from build123d import *

# Parameters (mm, degrees)
BOSS_EXTRUDE1_DEPTH = 12.7
SKETCH2_R           = 2.2479
CUT_EXTRUDE1_DEPTH  = 6.35
SKETCH3_W           = 25.4
SKETCH3_H           = 6.35
CUT_EXTRUDE2_DEPTH  = 6.35


with BuildPart() as part:
    # Sketch1 → Boss-Extrude1 (new body)
    with BuildSketch(Plane(origin=(0, 0, 0), x_dir=(1, 0, 0), z_dir=(0, 1, 0))):
        with BuildLine():
            ThreePointArc((0, -2.2479), (-2.2479, 0), (0, 2.2479))
            Line((0, 2.2479), (0, 3.175))
            ThreePointArc((0, 3.175), (-3.175, 0), (0, -3.175))
            Line((0, -3.175), (0, -2.2479))
        make_face()
        with BuildLine():
            ThreePointArc((0, -3.175), (-3.175, 0), (0, 3.175))
            Line((0, 3.175), (5.499261314, 3.175))
            ThreePointArc((5.499261314, 3.175), (-6.35, 0), (5.499261314, -3.175))
            Line((5.499261314, -3.175), (0, -3.175))
        make_face()
        with BuildLine():
            ThreePointArc((0, 2.2479), (1.589505333, 1.589505333), (2.2479, 0))
            Line((2.2479, 0), (3.175, 0))
            ThreePointArc((3.175, 0), (2.24506403, 2.24506403), (0, 3.175))
            Line((0, 3.175), (0, 2.2479))
        make_face()
        with BuildLine():
            Line((3.175, 0), (2.2479, 0))
            ThreePointArc((2.2479, 0), (1.589505333, -1.589505333), (0, -2.2479))
            Line((0, -2.2479), (0, -3.175))
            ThreePointArc((0, -3.175), (2.24506403, -2.24506403), (3.175, 0))
        make_face()
        with BuildLine():
            ThreePointArc((0, 3.175), (2.24506403, 2.24506403), (3.175, 0))
            Line((3.175, 0), (6.35, 0))
            ThreePointArc((6.35, 0), (6.133628997, 1.643500936), (5.499261314, 3.175))
            Line((5.499261314, 3.175), (0, 3.175))
        make_face()
        with BuildLine():
            Line((6.35, 0), (3.175, 0))
            ThreePointArc((3.175, 0), (2.24506403, -2.24506403), (0, -3.175))
            Line((0, -3.175), (5.499261314, -3.175))
            ThreePointArc((5.499261314, -3.175), (6.133628997, -1.643500936), (6.35, 0))
        make_face()
        with BuildLine():
            ThreePointArc((5.499261314, 3.175), (6.133628997, 1.643500936), (6.35, 0))
            Line((6.35, 0), (114.808, 0))
            ThreePointArc((114.808, 0), (115.024371003, 1.643500936), (115.658738686, 3.175))
            Line((115.658738686, 3.175), (5.499261314, 3.175))
        make_face()
        with BuildLine():
            Line((114.808, 0), (6.35, 0))
            ThreePointArc((6.35, 0), (6.133628997, -1.643500936), (5.499261314, -3.175))
            Line((5.499261314, -3.175), (115.658738686, -3.175))
            ThreePointArc((115.658738686, -3.175), (115.024371003, -1.643500936), (114.808, 0))
        make_face()
        with BuildLine():
            ThreePointArc((115.658738686, 3.175), (115.024371003, 1.643500936), (114.808, 0))
            Line((114.808, 0), (117.983, 0))
            ThreePointArc((117.983, 0), (118.91293597, 2.24506403), (121.158, 3.175))
            Line((121.158, 3.175), (115.658738686, 3.175))
        make_face()
        with BuildLine():
            Line((117.983, 0), (114.808, 0))
            ThreePointArc((114.808, 0), (115.024371003, -1.643500936), (115.658738686, -3.175))
            Line((115.658738686, -3.175), (121.158, -3.175))
            ThreePointArc((121.158, -3.175), (118.91293597, -2.24506403), (117.983, 0))
        make_face()
        with BuildLine():
            ThreePointArc((121.158, 3.175), (118.91293597, 2.24506403), (117.983, 0))
            Line((117.983, 0), (118.9101, 0))
            ThreePointArc((118.9101, 0), (119.568494667, 1.589505333), (121.158, 2.2479))
            Line((121.158, 2.2479), (121.158, 3.175))
        make_face()
        with BuildLine():
            Line((118.9101, 0), (117.983, 0))
            ThreePointArc((117.983, 0), (118.91293597, -2.24506403), (121.158, -3.175))
            ThreePointArc((121.158, -3.175), (123.40306403, -2.24506403), (124.333, 0))
            ThreePointArc((124.333, 0), (123.40306403, 2.24506403), (121.158, 3.175))
            Line((121.158, 3.175), (121.158, 2.2479))
            ThreePointArc((121.158, 2.2479), (122.747505333, 1.589505333), (123.4059, 0))
            ThreePointArc((123.4059, 0), (121.158, -2.2479), (118.9101, 0))
        make_face()
        with BuildLine():
            ThreePointArc((127.508, 0), (122.801500936, 6.133628997), (115.658738686, 3.175))
            Line((115.658738686, 3.175), (121.158, 3.175))
            ThreePointArc((121.158, 3.175), (123.40306403, 2.24506403), (124.333, 0))
            ThreePointArc((124.333, 0), (123.40306403, -2.24506403), (121.158, -3.175))
            Line((121.158, -3.175), (115.658738686, -3.175))
            ThreePointArc((115.658738686, -3.175), (122.801500936, -6.133628997), (127.508, 0))
        make_face()
    extrude(amount=BOSS_EXTRUDE1_DEPTH)

    # Sketch2 → Cut-Extrude1 (cut)
    # profile 1 of 6: a face of its own
    with BuildSketch(Plane.XZ):
        with BuildLine():
            Line((12.7, -3.175), (12.7, 3.175))
            Line((12.7, 3.175), (5.499261314, 3.175))
            ThreePointArc((5.499261314, 3.175), (6.133628997, 1.643500936), (6.35, 0))
            ThreePointArc((6.35, 0), (6.133628997, -1.643500936), (5.499261314, -3.175))
            Line((5.499261314, -3.175), (12.7, -3.175))
        make_face()
    # profile 2 of 6: a face of its own
    with BuildSketch(Plane.XZ):
        with BuildLine():
            ThreePointArc((6.35, 0), (6.133628997, 1.643500936), (5.499261314, 3.175))
            Line((5.499261314, 3.175), (2.654111014, 3.175))
            Line((2.654111014, 3.175), (2.654111014, -3.175))
            Line((2.654111014, -3.175), (5.499261314, -3.175))
            ThreePointArc((5.499261314, -3.175), (6.133628997, -1.643500936), (6.35, 0))
        make_face()
    # profile 3 of 6: a face of its own
    with BuildSketch(Plane.XZ):
        with BuildLine():
            Line((2.654111014, 3.175), (5.499261314, 3.175))
            ThreePointArc((5.499261314, 3.175), (-6.35, 0), (5.499261314, -3.175))
            Line((5.499261314, -3.175), (2.654111014, -3.175))
            Line((2.654111014, -3.175), (2.654111014, 3.175))
        make_face()
        with Locations(Location((0, 0, 0), (0, 0, 270))):
            Circle(SKETCH2_R, mode=Mode.SUBTRACT)
    # profile 4 of 6: a face of its own
    with BuildSketch(Plane.XZ):
        with BuildLine():
            ThreePointArc((127.508, 0), (122.801500936, 6.133628997), (115.658738686, 3.175))
            Line((115.658738686, 3.175), (118.641772853, 3.175))
            Line((118.641772853, 3.175), (118.641772853, -3.175))
            Line((118.641772853, -3.175), (115.658738686, -3.175))
            ThreePointArc((115.658738686, -3.175), (122.801500936, -6.133628997), (127.508, 0))
        make_face()
        with Locations(Location((121.158, 0, 0), (0, 0, 270))):
            Circle(SKETCH2_R, mode=Mode.SUBTRACT)
    # profile 5 of 6: a face of its own
    with BuildSketch(Plane.XZ):
        with BuildLine():
            Line((115.658738686, 3.175), (108.458, 3.175))
            Line((108.458, 3.175), (108.458, -3.175))
            Line((108.458, -3.175), (115.658738686, -3.175))
            ThreePointArc((115.658738686, -3.175), (114.808, 0), (115.658738686, 3.175))
        make_face()
    # profile 6 of 6: a face of its own
    with BuildSketch(Plane.XZ):
        with BuildLine():
            Line((118.641772853, 3.175), (115.658738686, 3.175))
            ThreePointArc((115.658738686, 3.175), (114.808, 0), (115.658738686, -3.175))
            Line((115.658738686, -3.175), (118.641772853, -3.175))
            Line((118.641772853, -3.175), (118.641772853, 3.175))
        make_face()
    extrude(amount=-CUT_EXTRUDE1_DEPTH, mode=Mode.SUBTRACT)

    # Sketch3 → Cut-Extrude2 (cut)
    with BuildSketch(Plane.XZ):
        with Locations((60.579, 0)):
            Rectangle(SKETCH3_W, SKETCH3_H)
    extrude(amount=-CUT_EXTRUDE2_DEPTH, mode=Mode.SUBTRACT)


solid = part.part
Model file for the job. Use its own axes, mm. A direction names the side the tool comes from. Give positions to 0.01 mm unless a question says otherwise; leave off trailing zeros. Order: outer loops, then holes, each group sorted by start corner. A loop starts at its lowest first (then second) coordinate and runs counter-clockwise, first axis right, second up. Notation, with made-up numbers: (4, 78) -> (18, 78) arc R31 ccw to (18, 113) -> close; hole circle Ø2 at (-6, 67). An arc over 180 degrees is marked (long way). Use CSV: the item, a comma, the result in double quotes.
1. Band-saw the part on B-B, the plane z = 5. Give the cut face in (x, y), then the cut area to 3 significant figures.
Outcome:
outline,"(-3.91, 6.35) -> (3.91, 6.35) -> (3.91, 12.7) -> (-3.91, 12.7) -> close; (117.24, 6.35) -> (125.07, 6.35) -> (125.07, 12.7) -> (117.24, 12.7) -> close"
area,"99.4 mm²"
2. Band-saw the part on C-C, the plane x = 11.5. Give the cut face in (y, z) (3 decimals).
Outcome:
outline,"(6.35, -3.175) -> (12.7, -3.175) -> (12.7, 3.175) -> (6.35, 3.175) -> close"
3. Band-saw the part on D-D, the plane x = 32. Give the cut face in (y, z) (3 decimals), then the cut area to 3 significant figures.
Outcome:
outline,"(0, -3.175) -> (12.7, -3.175) -> (12.7, 3.175) -> (0, 3.175) -> close"
area,"80.6 mm²"
4. Band-saw the part on A-A, the plane y = 9. Give the cut face in (x, z) (3 decimals).
Outcome:
outline,"(5.499, -3.175) -> (115.659, -3.175) arc R6.35 ccw (long way) to (115.659, 3.175) -> (5.499, 3.175) arc R6.35 ccw (long way) to start; hole circle Ø4.496 at (0, 0); hole circle Ø4.496 at (121.158, 0)"
5. Drop flat-ended pins along their axis: pin 1 (5 mm diameter, centred on x = 42.5, y = 8.5, fed in from -Z) (3 decimals); pin 2 (3 mm diameter, centred on y = 2, z = 1.5, fed in from -X); pin 3 (4 mm diameter, centred on y = 4, z = 2.5, fed in from +X); pin 4 (1 mm diameter, centred on x = 47, z = -5, fed in from -Y). Give the stop position or say it passes through.
Outcome:
pin 1,"z = -3.175"
pin 2,"x = 12.7"
pin 3,"x = 108.46"
pin 4,"through"
6. Mould opens along X. For faces 5 (the flat face through (108.458, 3, 0)), 6 (the cylindrical face through (-6.346, 9.481, -0.233)), 7 (the flat face through (30, 0, 0)) say: +X half, -X half, draft (parallel to the pull), parting line (faces both ways), or undercut.
Outcome:
face 5,"+X half"
face 6,"undercut"
face 7,"draft"
7. Drill centre lines: line 1 along X through (y, z) = (5.75, -1.5); line 2 along X through (y, z) = (12.25, -1); line 3 along X through (y, z) = (8.5, -0.75). Where is each one in solid material? Low to high. Write a range as from..to.
Outcome:
line 1,"12.7..47.88, 73.28..108.46"
line 2,"-6.27..-2.01, 2.01..119.14, 123.17..127.43"
line 3,"-6.31..-2.12, 2.12..119.04, 123.28..127.46"
8. 3-axis set-ups, long thin cutter, end or side, ignore diameter. For faces 1 (the flat face through (12.7, 3, 0)), 2 (the flat face through (61, 8, -3.175)), 3 (the flat face through (118, 6.35, 0)), 4 (the flat face through (73.279, 3, 0)): which of +Z, -Z, +X, -X, +Y, -Y reach the whole face in a straight line?
Outcome:
face 1,"+Z, -Z, -X, -Y"
face 2,"-Z, +Y, -Y"
face 3,"+Z, -Z, +X, -Y"
face 4,"+Z, -Z, -Y"
